Design review of the part built by this model. Coordinates are the model's own, in mm. Face numbers are marked on the shaded views. A direction names the side the tool comes from. Coordinates: 2 decimals unless noted, no trailing zeros. Write each loop counter-clockwise with the first axis right and the second up, starting at its lowest first coordinate (ties: lowest second). Pieces come first, ordered by that corner, then holes.
Q1. Machinability: for the marked faces 1 and 2, which of the approach directions +Z, -Z, +X, -X, +Y, -Y give a long, thin tool a straight path to every point of the face, cutting with its end or side? Answer none if there is none.
Q2. Take a section at A-A (z = 130). Give the boundary of the cut face in (x, y).
Q3. Take a section at D-D (x = 32). State how many separate pieces and enclosed holes the cut face has, and give its area (4 significant figures).
Q4. Insertion check: pin 1 (10 mm diameter, centred on x = -96, z = 52, fed in from -Y); pin 2 (9 mm diameter, centred on y = 147.5, z = -140.5, fed in from -X); pin 3 (2 mm diameter, centred on x = 75.5, z = -101.5, fed in from +Y). Each pin has a flat end and moves straight along its axis. Give the tip position at first contact, or say it passes through.
Q5. For probe 1 along Z at (x, y) = (37.5, 112); probe 2 along Z at (x, y) = (-43.5, 21); probe 3 along Z at (x, y) = (109, 150.5), list the stretches that pass through material, from the lowest coordinate up.
Q6. Take a section at B-B (y = 198). Give the boundary of the cut face in (x, z).
Q7. Mouldability with a two-part tool opening along Z and no side actions: class the marked faces 3, 4 and 5 as pulls with the +Z half, pulls with the -Z half, needs draft (parallel to the pull), parting line crosses it, or undercut.
Q8. Take a section at C-C (z = -100.5). Give the boundary of the cut face in (x, y).
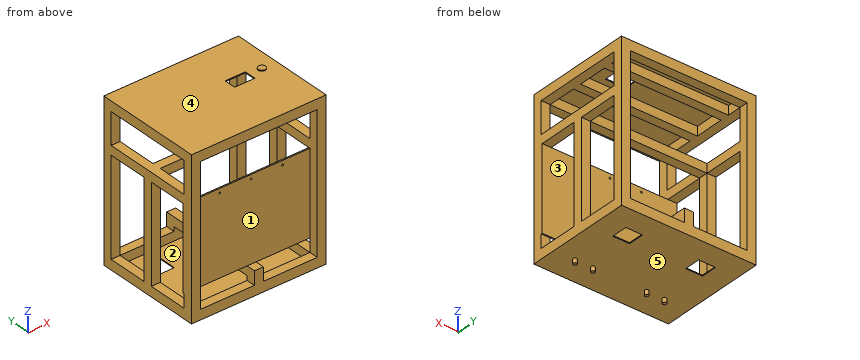
```python
from build123d import *

# Parameters (mm, degrees)
SKETCH_1_W          = 300
SKETCH_1_H          = 345
EXTRUDE_1_DEPTH     = 240
SKETCH_2_W          = 260
SKETCH_2_H          = 305
CUT_EXTRUDE_1_DEPTH = 240
SKETCH_3_W          = 260
SKETCH_3_H          = 200
CUT_EXTRUDE_2_DEPTH = 345
SKETCH_4_W          = 305
SKETCH_4_H          = 200
CUT_EXTRUDE_3_DEPTH = 345
SKETCH_5_W          = 20
SKETCH_5_H          = 240
EXTRUDE_2_DEPTH     = 20
SKETCH_6_W          = 20
SKETCH_6_H          = 240
EXTRUDE_3_DEPTH     = 20
SKETCH_10_W         = 20
SKETCH_10_H         = 240
EXTRUDE_7_DEPTH     = 50
SKETCH_11_W         = 20
SKETCH_11_H         = 200
CUT_EXTRUDE_4_DEPTH = 50
SKETCH_12_W         = 20
SKETCH_12_H         = 20
EXTRUDE_8_DEPTH     = 240
SKETCH_13_W         = 20
SKETCH_13_H         = 20
EXTRUDE_9_DEPTH     = 300
SKETCH_14_W         = 300
SKETCH_14_H         = 185
EXTRUDE_10_DEPTH    = 3
SKETCH_15_R         = 2.05
CUT_EXTRUDE_5_DEPTH = 3
SKETCH_16_W         = 215
SKETCH_16_H         = 20
EXTRUDE_11_DEPTH    = 20
SKETCH_17_W         = 215
SKETCH_17_H         = 20
EXTRUDE_12_DEPTH    = 20
SKETCH_18_W         = 300
SKETCH_18_H         = 240
EXTRUDE_13_DEPTH    = 2
SKETCH_20_W         = 300
SKETCH_20_H         = 240
EXTRUDE_14_DEPTH    = 2
SKETCH_21_R         = 8.165036004
EXTRUDE_15_DEPTH    = 2
SKETCH_22_W         = 300
SKETCH_22_H         = 20
EXTRUDE_16_DEPTH    = 22
SKETCH_24_W         = 45
SKETCH_24_H         = 26
CUT_EXTRUDE_6_DEPTH = 2
SKETCH_25_W         = 37.5
SKETCH_25_H         = 35.5
CUT_EXTRUDE_7_DEPTH = 2
SKETCH_26_W         = 37.5
SKETCH_26_H         = 35.5
CUT_EXTRUDE_8_DEPTH = 2
SKETCH_27_R         = 4
EXTRUDE_17_DEPTH    = 10
SKETCH_28_R         = 4
EXTRUDE_18_DEPTH    = 10


with BuildPart() as part:
    # 草图1 → 凸台-拉伸1 (new body)
    with BuildSketch(Plane(origin=(0, 0, 0), x_dir=(1, 0, 0), z_dir=(0, 1, 0))):
        Rectangle(SKETCH_1_W, SKETCH_1_H)
    extrude(amount=EXTRUDE_1_DEPTH)

    # 草图2 → 切除-拉伸1 (cut)
    with BuildSketch(Plane(origin=(0, 240, 0), x_dir=(1, 0, 0), z_dir=(0, 1, 0))):
        Rectangle(SKETCH_2_W, SKETCH_2_H)
    extrude(amount=-CUT_EXTRUDE_1_DEPTH, mode=Mode.SUBTRACT)

    # 草图3 → 切除-拉伸2 (cut)
    with BuildSketch(Plane.XY.offset(172.5)):
        with Locations((0, 120)):
            Rectangle(SKETCH_3_W, SKETCH_3_H)
    extrude(amount=-CUT_EXTRUDE_2_DEPTH, mode=Mode.SUBTRACT)

    # 草图4 → 切除-拉伸3 (cut)
    with BuildSketch(Plane.ZY.offset(150)):
        with Locations((0, 120)):
            Rectangle(SKETCH_4_W, SKETCH_4_H)
    extrude(amount=-CUT_EXTRUDE_3_DEPTH, mode=Mode.SUBTRACT)

    # 草图5 → 凸台-拉伸2 (add)
    with BuildSketch(Plane(origin=(150, 0, 0), x_dir=(0, 0, -1), z_dir=(1, 0, 0))):
        with Locations((-72.5, 120)):
            Rectangle(SKETCH_5_W, SKETCH_5_H)
    extrude(amount=-EXTRUDE_2_DEPTH)

    # 草图6 → 凸台-拉伸3 (add)
    with BuildSketch(Plane.ZY.offset(150)):
        with Locations((72.5, 120)):
            Rectangle(SKETCH_6_W, SKETCH_6_H)
    extrude(amount=-EXTRUDE_3_DEPTH)

    # 草图10 → 凸台-拉伸7 (add)
    with BuildSketch(Plane(origin=(0, 0, -172.5), x_dir=(-1, 0, 0), z_dir=(0, 0, -1))):
        with Locations((0, 120)):
            Rectangle(SKETCH_10_W, SKETCH_10_H)
    extrude(amount=-EXTRUDE_7_DEPTH)

    # 草图11 → 切除-拉伸4 (cut)
    with BuildSketch(Plane(origin=(0, 0, -172.5), x_dir=(-1, 0, 0), z_dir=(0, 0, -1))):
        with Locations((0, 120)):
            Rectangle(SKETCH_11_W, SKETCH_11_H)
    extrude(amount=-CUT_EXTRUDE_4_DEPTH, mode=Mode.SUBTRACT)

    # 草图12 → 凸台-拉伸8 (add)
    with BuildSketch(Plane(origin=(0, 240, 0), x_dir=(1, 0, 0), z_dir=(0, 1, 0))):
        with Locations((0, 132.5)):
            Rectangle(SKETCH_12_W, SKETCH_12_H)
    extrude(amount=-EXTRUDE_8_DEPTH)

    # 草图13 → 凸台-拉伸9 (add)
    with BuildSketch(Plane(origin=(150, 0, 0), x_dir=(0, 0, -1), z_dir=(1, 0, 0))):
        with Locations((-72.5, 120)):
            Rectangle(SKETCH_13_W, SKETCH_13_H)
    extrude(amount=-EXTRUDE_9_DEPTH)

    # 草图14 → 凸台-拉伸10 (add)
    with BuildSketch(Plane(origin=(0, 20, 0), x_dir=(1, 0, 0), z_dir=(0, 1, 0))):
        with Locations((0, 30)):
            Rectangle(SKETCH_14_W, SKETCH_14_H)
    extrude(amount=EXTRUDE_10_DEPTH)

    # 草图15 → 切除-拉伸5 (cut)
    with BuildSketch(Plane(origin=(0, 23, 0), x_dir=(1, 0, 0), z_dir=(0, 1, 0))):
        with Locations(Location((-70.947060375, -52.987042074, 0), (0, 0, 270))):
            Circle(SKETCH_15_R)
        with Locations(Location((-0.947060375, -52.987042074, 0), (0, 0, 270))):
            Circle(SKETCH_15_R)
        with Locations(Location((69.052939625, -52.987042074, 0), (0, 0, 270))):
            Circle(SKETCH_15_R)
    extrude(amount=-CUT_EXTRUDE_5_DEPTH, mode=Mode.SUBTRACT)

    # 草图16 → 凸台-拉伸11 (add)
    with BuildSketch(Plane(origin=(150, 0, 0), x_dir=(0, 0, -1), z_dir=(1, 0, 0))):
        with Locations((45, 120)):
            Rectangle(SKETCH_16_W, SKETCH_16_H)
    extrude(amount=-EXTRUDE_11_DEPTH)

    # 草图17 → 凸台-拉伸12 (add)
    with BuildSketch(Plane.ZY.offset(150)):
        with Locations((-45, 120)):
            Rectangle(SKETCH_17_W, SKETCH_17_H)
    extrude(amount=-EXTRUDE_12_DEPTH)

    # 草图18 → 凸台-拉伸13 (add)
    with BuildSketch(Plane.XY.offset(172.5)):
        with Locations((0, 120)):
            Rectangle(SKETCH_18_W, SKETCH_18_H)
    extrude(amount=EXTRUDE_13_DEPTH)

    # 草图20 → 凸台-拉伸14 (add)
    with BuildSketch(Plane(origin=(0, 0, -172.5), x_dir=(-1, 0, 0), z_dir=(0, 0, -1))):
        with Locations((0, 120)):
            Rectangle(SKETCH_20_W, SKETCH_20_H)
    extrude(amount=EXTRUDE_14_DEPTH)

    # 草图21 → 凸台-拉伸15 (add)
    with BuildSketch(Plane.XY.offset(174.5)):
        with Locations((116.249294112, 134.333303452)):
            Circle(SKETCH_21_R)
    extrude(amount=EXTRUDE_15_DEPTH)

    # 草图22 → 凸台-拉伸16 (add)
    with BuildSketch(Plane.XY.offset(174.5)):
        with Locations((0, 178.667130527)):
            Rectangle(SKETCH_22_W, SKETCH_22_H)
        with Locations((0, 93.667130527)):
            Rectangle(SKETCH_22_W, SKETCH_22_H)
    extrude(amount=-EXTRUDE_16_DEPTH)

    # 草图24 → 切除-拉伸6 (cut)
    with BuildSketch(Plane.XY.offset(174.5)):
        with Locations((65.114949377, 131.614411481)):
            Rectangle(SKETCH_24_W, SKETCH_24_H)
    extrude(amount=-CUT_EXTRUDE_6_DEPTH, mode=Mode.SUBTRACT)

    # 草图25 → 切除-拉伸7 (cut)
    with BuildSketch(Plane(origin=(0, 0, -174.5), x_dir=(-1, 0, 0), z_dir=(0, 0, -1))):
        with Locations((81.25, 172.25)):
            Rectangle(SKETCH_25_W, SKETCH_25_H)
    extrude(amount=-CUT_EXTRUDE_7_DEPTH, mode=Mode.SUBTRACT)

    # 草图26 → 切除-拉伸8 (cut)
    with BuildSketch(Plane(origin=(0, 0, -174.5), x_dir=(-1, 0, 0), z_dir=(0, 0, -1))):
        with Locations((-81.25, 172.25)):
            Rectangle(SKETCH_26_W, SKETCH_26_H)
    extrude(amount=-CUT_EXTRUDE_8_DEPTH, mode=Mode.SUBTRACT)

    # 草图27 → 凸台-拉伸17 (add)
    with BuildSketch(Plane(origin=(0, 0, -174.5), x_dir=(-1, 0, 0), z_dir=(0, 0, -1))):
        with Locations((-104.657434269, 57.050217573)):
            Circle(SKETCH_27_R)
        with Locations((-64.657434269, 57.050217573)):
            Circle(SKETCH_27_R)
    extrude(amount=EXTRUDE_17_DEPTH)

    # 草图28 → 凸台-拉伸18 (add)
    with BuildSketch(Plane(origin=(0, 0, -174.5), x_dir=(-1, 0, 0), z_dir=(0, 0, -1))):
        with Locations((54.161932501, 57.839316769)):
            Circle(SKETCH_28_R)
        with Locations((94.161932501, 57.839316769)):
            Circle(SKETCH_28_R)
    extrude(amount=EXTRUDE_18_DEPTH)


solid = part.part
```
Response:
1. face 1: -Y
1. face 2: none
2. outline: (-150, 0) - (-130, 0) - (-130, 20) - (-150, 20) - close; (-150, 220) - (-130, 220) - (-130, 240) - (-150, 240) - close; (130, 0) - (150, 0) - (150, 20) - (130, 20) - close; (130, 220) - (150, 220) - (150, 240) - (130, 240) - close
3. separate pieces: 4
3. enclosed holes: 0
3. area: 4,315 mm2
4. pin 1: stops at y = 20
4. pin 2: stops at x = -10
4. pin 3: stops at y = 23
5. probe 1: z = -174.5 to -172.5, 62.5 to 82.5, 172.5 to 174.5
5. probe 2: z = -174.5 to -172.5, -122.5 to 62.5, 172.5 to 174.5
5. probe 3: z = -174.5 to -172.5, 172.5 to 174.5
6. outline: (-150, -174.5) - (150, -174.5) - (150, -152.5) - (130, -152.5) - (130, -172.5) - (-130, -172.5) - (-130, -152.5) - (-150, -152.5) - close; (-150, 62.5) - (-130, 62.5) - (-130, 82.5) - (-150, 82.5) - close; (-150, 152.5) - (-130, 152.5) - (-130, 172.5) - (130, 172.5) - (130, 152.5) - (150, 152.5) - (150, 174.5) - (-150, 174.5) - close; (-10, -142.5) - (10, -142.5) - (10, -122.5) - (-10, -122.5) - close; (130, 62.5) - (150, 62.5) - (150, 82.5) - (130, 82.5) - close
7. face 3: undercut
7. face 4: pulls with the +Z half
7. face 5: pulls with the -Z half
8. outline: (-150, 0) - (-130, 0) - (-130, 20) - (130, 20) - (130, 0) - (150, 0) - (150, 23) - (-150, 23) - close; (-150, 110) - (-130, 110) - (-130, 130) - (-150, 130) - close; (-150, 220) - (-130, 220) - (-130, 240) - (-150, 240) - close; (130, 110) - (150, 110) - (150, 130) - (130, 130) - close; (130, 220) - (150, 220) - (150, 240) - (130, 240) - close
